Autodesk Inventor part; units mm, degrees
ref_plane "YZ Plane" through (0, 0, 0) normal (1, 0, 0) x (0, 1, 0)
ref_plane "XZ Plane" through (0, 0, 0) normal (0, 1, 0) x (-1, 0, 0)
ref_plane "XY Plane" through (0, 0, 0) normal (0, 0, 1) x (1, 0, 0)
sketch "Sketch1" plane through (0, 0, 0) normal (0, 1, 0) x (-1, 0, 0)
  line L0 (0, 0) -> (-54.3, 0)
  line L1 (-54.3, 0) -> (-54.3, -65.9)
  line L2 (-54.3, -65.9) -> (0, -65.9)
  line L3 (0, -65.9) -> (0, 0)
  dimension "d0" = 54.3
  dimension "d1" = 65.9
extrude "Extrusion1" add sketch "Sketch1" along normal blind 1.6
sketch "Sketch2" plane through (0, 1.6, 0) normal (0, 1, 0) x (1, 0, 0)
  line L0 (0, 65.9) -> (0, 0)
  line L1 (54.3, 65.9) -> (0, 65.9)
  line L2 (54.3, 0) -> (54.3, 65.9)
  line L3 (0, 0) -> (54.3, 0)
  point P0 (4.2, 61.6)
  point P1 (50.3, 61.7)
  point P2 (4, 4.3)
  dimension "d4" = 4.2
  dimension "d5" = 4.3
  dimension "d6" = 4
  dimension "d7" = 4.2
  dimension "d8" = 4
  dimension "d9" = 4.3
hole "Hole1" at (4.2, 1.6, -61.6) at (50.3, 1.6, -61.7) at (4, 1.6, -4.3) direction (0, -1, 0) diameter 3.175 end through all
sketch "Sketch3" plane through (0, 1.6, 0) normal (0, 1, 0) x (1, 0, 0)
  line L0 (53.4872, 53.8448) -> (53.4872, 2.8448)
  line L1 (30.4872, 2.8448) -> (30.4872, 52.8828)
  line L2 (0, 0) -> (54.3, 0)
  line L3 (54.3, 0) -> (54.3, 65.9)
  line L4 (33.0272, 52.8828) -> (33.0272, 2.8448)
  line L5 (50.9472, 53.8448) -> (50.9472, 2.8448)
  line L6 (30.4872, 52.8828) -> (33.0272, 52.8828)
  line L7 (50.9472, 53.8448) -> (53.4872, 53.8448)
  line L8 (53.4872, 2.8448) -> (50.9472, 2.8448)
  line L9 (33.0272, 2.8448) -> (30.4872, 2.8448)
  dimension "d17" = 23
  dimension "d18" = 51
  dimension "d20" = 0.8128
  dimension "d21" = 2.54
  dimension "d22" = 2.54
extrude "Extrusion2" add sketch "Sketch3" along normal blind 5.08
sketch "Sketch4" plane through (0, 6.68, 0) normal (0, 1, 0) x (1, 0, 0)
  line L0 (30.4872, 52.8828) -> (30.4872, 2.8448)
  line L1 (30.4872, 2.8448) -> (33.0272, 2.8448)
  line L2 (33.0272, 2.8448) -> (33.0272, 52.8828)
  line L3 (33.0272, 52.8828) -> (30.4872, 52.8828)
  line L4 (53.4872, 2.8448) -> (53.4872, 53.8448)
  line L5 (50.9472, 53.8448) -> (50.9472, 2.8448)
  line L6 (50.9472, 2.8448) -> (53.4872, 2.8448)
  line L7 (53.4872, 53.8448) -> (50.9472, 53.8448)
  line L8 (30.4872, 52.8828) -> (30.4872, 2.8448)
  line L9 (30.4872, 52.8828) -> (53.4872, 52.8828)
  line L10 (53.4872, 52.8828) -> (53.4872, 2.8448)
  line L11 (53.4872, 2.8448) -> (30.4872, 2.8448)
  line L12 (30.4872, 2.8448) -> (30.4872, 52.8828)
  point P0 (0, 0)
extrude "Extrusion3" add sketch "Sketch4" along normal blind 1.6 contours L3 L2 L1 L0 | L9 L5 L11 L2 | L9 L4 L6 L5
sketch "Sketch5" plane through (0, 8.28, 0) normal (0, 1, 0) x (1, 0, 0)
  line L0 (45.4872, 47.7) -> (53.4872, 47.7)
  line L1 (53.4872, 47.7) -> (53.4872, 39.7)
  line L2 (53.4872, 39.7) -> (45.4872, 39.7)
  line L3 (45.4872, 39.7) -> (45.4872, 47.7)
  line L4 (53.4872, 2.8448) -> (53.4872, 52.8828)
  line L5 (53.4872, 52.8828) -> (30.4872, 52.8828)
  line L6 (0, 0) -> (54.3, 0)
  line L7 (30.4872, 52.8828) -> (30.4872, 2.8448)
  line L8 (30.4872, 2.8448) -> (53.4872, 2.8448)
  line L9 (53.4872, 2.8448) -> (53.4872, 52.8828)
  line L10 (53.4872, 52.8828) -> (30.4872, 52.8828)
  dimension "d27" = 8
  dimension "d28" = 8
  dimension "d61" = 39.7
extrude "Extrusion4" add sketch "Sketch5" along normal blind 6.4 contours L0 L1 L2 L3
sketch "Sketch7" plane through (0, 1.6, 0) normal (0, 1, 0) x (1, 0, 0)
  line L0 (1.016, 48.6) -> (6.096, 48.6)
  line L1 (6.096, 48.6) -> (6.096, 41)
  line L2 (6.096, 41) -> (1.016, 41)
  line L3 (1.016, 41) -> (1.016, 48.6)
  line L4 (54.3, 65.9) -> (0, 65.9)
  line L5 (0, 65.9) -> (0, 0)
  dimension "d32" = 5.08
  dimension "d33" = 7.6
  dimension "d34" = 17.3
  dimension "d35" = 1.016
extrude "Extrusion5" add sketch "Sketch7" along normal blind 2.5
sketch "Sketch8" plane through (0, 1.6, 0) normal (0, 1, 0) x (1, 0, 0)
  line L0 (11.4, 65.011) -> (17.268, 65.011)
  line L1 (17.268, 65.011) -> (17.268, 57.01)
  line L2 (17.268, 57.01) -> (11.4, 57.01)
  line L3 (11.4, 57.01) -> (11.4, 65.011)
  line L4 (0, 65.9) -> (0, 0)
  line L5 (54.3, 65.9) -> (0, 65.9)
  line L6 (20.5192, 65.011) -> (26.4, 65.011)
  line L7 (26.4, 65.011) -> (26.4, 57.01)
  line L8 (26.4, 57.01) -> (20.5192, 57.01)
  line L9 (20.5192, 57.01) -> (20.5192, 65.011)
  dimension "d39" = 8.001
  dimension "d40" = 11.4
  dimension "d41" = 0.889
  dimension "d43" = 8.001
  dimension "d44" = 3.2512
  dimension "d45" = 0.889
  dimension "d60" = 15
extrude "Extrusion6" add sketch "Sketch8" against normal blind 8.1
sketch "Sketch9" plane through (0, 1.6, 0) normal (0, 1, 0) x (1, 0, 0)
  line L0 (8.6868, 53.454) -> (28.6584, 53.454)
  line L1 (28.6584, 53.454) -> (28.6584, 0.6858)
  line L2 (28.6584, 0.6858) -> (8.6868, 0.6858)
  line L3 (8.6868, 0.6858) -> (8.6868, 53.454)
  line L4 (54.3, 65.9) -> (0, 65.9)
  line L5 (30.4872, 52.8828) -> (30.4872, 2.8448)
  line L6 (0, 65.9) -> (0, 0)
  line L7 (0, 0) -> (54.3, 0)
  dimension "d48" = 12.446
  dimension "d49" = 1.8288
  dimension "d50" = 8.6868
  dimension "d51" = 0.6858
extrude "Extrusion7" add sketch "Sketch9" along normal up to surface (6.68 mm away)
sketch "Sketch10" plane through (0, 0, 0) normal (0, -1, 0) x (1, 0, 0)
  line L0 (42.5398, -21.577) -> (24.1808, -21.577)
  line L1 (24.1808, -21.577) -> (24.1808, -12.2936)
  line L2 (24.1808, -12.2936) -> (42.5398, -12.2936)
  line L3 (42.5398, -12.2936) -> (42.5398, -21.577)
  line L4 (54.3, -65.9) -> (0, -65.9)
  line L5 (54.3, 0) -> (54.3, -65.9)
  line L6 (0, -65.9) -> (0, 0)
  line L7 (0, 0) -> (54.3, 0)
  dimension "d54" = 44.323
  dimension "d55" = 11.7602
  dimension "d56" = 24.1808
  dimension "d57" = 12.2936
extrude "Extrusion8" add sketch "Sketch10" along normal blind 1.016 contours L0 L1 L2 L3
properties part number "PCB"
Here's how the part is built. I have some questions about the finished solid (model axes, mm). A direction names the side the tool comes from. Coordinates: 2 decimals unless noted, no trailing zeros. Write each loop counter-clockwise with the first axis right and the second up, starting at its lowest first coordinate (ties: lowest second). Pieces come first, ordered by that corner, then holes.
Item 1: I want a section at C-C on z = -46.5. Write out the boundary of the cut face in (x, y), and give its area (3 significant figures).
Item 2: Will these pins go through, and if not, where does the flat tip stop? pin 1 (12 mm diameter, centred on y = -4, z = -58, fed in from +X); pin 2 (4 mm diameter, centred on x = 44.5, y = 5, fed in from -Z); pin 3 (5 mm diameter, centred on x = 11, y = -3.5, fed in from -Z); pin 4 (2 mm diameter, centred on y = 5.5, z = -28, fed in from -X).
Item 3: I want a section at A-A on y = -5. Write out the boundary of the cut face in (x, z).
Item 4: If we mould it in two halves opening along Z, with no side actions, what happens to faces 5 (the cylindrical face through (3.723, 0.789, -60.086)), 6 (the flat face through (50, 11, -39.7)), 7 (the flat face through (11.4, -3, -61))? For each: +Z half, -Z half, draft (parallel to the pull), parting line (faces both ways), or undercut.
Item 5: I want a section at D-D on x = 35.5. Write out the boundary of the cut face in (y, z).
Item 6: On a 3-axis mill with a long thin cutter (end or side, diameter ignored), from which of +Z, -Z, +X, -X, +Y, -Y can I reach the whole of each face in a straight line? I mean faces 1 (the flat face through (14, -3, -57.01)), 2 (the flat face through (30.487, 5, -28)), 3 (the flat face through (19, 5, -53.454)), 4 (the flat face through (14, -3, -65.011)). Say none if no direction works.
Item 7: I want a section at B-B on z = -4.3. Write out the boundary of the cut face in (x, y), and give its area (3 significant figures).
Item 8: If I drill on line 1 (X direction, y = 0.6, z = -61.6); line 2 (X direction, y = 5.75, z = -49); line 3 (Z direction, x = 4.2, y = 1.25), over which ranges is the centre line in solid material (lowest first)?
Findings below:
1. outline: (0, 0) - (54.3, 0) - (54.3, 1.6) - (53.49, 1.6) - (53.49, 14.68) - (45.49, 14.68) - (45.49, 8.28) - (30.49, 8.28) - (30.49, 1.6) - (28.66, 1.6) - (28.66, 8.28) - (8.69, 8.28) - (8.69, 1.6) - (6.1, 1.6) - (6.1, 4.1) - (1.02, 4.1) - (1.02, 1.6) - (0, 1.6) - close; hole (33.03, 1.6) - (50.95, 1.6) - (50.95, 6.68) - (33.03, 6.68) - close
1. area: 347 mm2
2. pin 1: stops at x = 54.3
2. pin 2: stops at z = -52.88
2. pin 3: stops at z = -65.01
2. pin 4: stops at x = 8.69
3. outline: (11.4, -65.01) - (17.27, -65.01) - (17.27, -57.01) - (11.4, -57.01) - close; (20.52, -65.01) - (26.4, -65.01) - (26.4, -57.01) - (20.52, -57.01) - close
4. face 5: undercut
4. face 6: +Z half
4. face 7: draft
5. outline: (-1.02, -21.58) - (0, -21.58) - (0, -65.9) - (1.6, -65.9) - (1.6, 0) - (0, 0) - (0, -12.29) - (-1.02, -12.29) - close; (6.68, -52.88) - (8.28, -52.88) - (8.28, -2.84) - (6.68, -2.84) - close
6. face 1: +Z, +X, -X, -Y
6. face 2: +Z, -Z, +Y
6. face 3: -Z, -X, +Y
6. face 4: -Z, +X, -X, -Y
7. outline: (0, 0) - (2.41, 0) - (2.41, 1.6) - (0, 1.6) - close; (5.59, 0) - (54.3, 0) - (54.3, 1.6) - (53.49, 1.6) - (53.49, 8.28) - (30.49, 8.28) - (30.49, 1.6) - (28.66, 1.6) - (28.66, 8.28) - (8.69, 8.28) - (8.69, 1.6) - (5.59, 1.6) - close; hole (33.03, 1.6) - (50.95, 1.6) - (50.95, 6.68) - (33.03, 6.68) - close
7. area: 278 mm2
8. line 1: x = 0 to 2.61, 5.79 to 48.72, 51.88 to 54.3
8. line 2: x = 8.69 to 28.66, 30.49 to 33.03, 50.95 to 53.49
8. line 3: z = -65.9 to -63.19, -60.01 to -5.87, -2.73 to 0
